```python
from build123d import *

# Parameters (mm, degrees)
SKETCH_1_W             = 80
SKETCH_1_H             = 60
SKETCH_1_W_2           = 78.6
SKETCH_1_H_2           = 58.6
EXTRUDE_1_DEPTH        = 1000
CUT_EXTRUDE_1_REACH    = 1004.597
SKETCH_2_W             = 40
SKETCH_2_H             = 40
PATTERN_LINEAR_1_COUNT = 5
PATTERN_LINEAR_1_PITCH = 200


with BuildPart() as part:
    # 스케치1 → 보스-돌출1 (new body)
    with BuildSketch(Plane.XY):
        Rectangle(SKETCH_1_W, SKETCH_1_H)
        Rectangle(SKETCH_1_W_2, SKETCH_1_H_2, mode=Mode.SUBTRACT)
    extrude(amount=EXTRUDE_1_DEPTH)

    # 스케치2 → 컷-돌출1 (cut, up to next)
    with BuildSketch(Plane(origin=(0, 30, 0), x_dir=(1, 0, 0), z_dir=(0, 1, 0)), mode=Mode.PRIVATE) as cut_extrude_1_sk1:
        with Locations((0, -40)):
            Rectangle(SKETCH_2_W, SKETCH_2_H)
    cut_extrude_1_tool1 = extrude(cut_extrude_1_sk1.sketch, amount=-CUT_EXTRUDE_1_REACH, mode=Mode.PRIVATE) & part.part
    cut_extrude_1 = cut_extrude_1_tool1.solids().sort_by_distance((0, 30, 40))[0]
    add(cut_extrude_1, mode=Mode.SUBTRACT)

    # 선형 패턴1: 컷-돌출1 ×5
    with Locations(*[(0, 0, i * PATTERN_LINEAR_1_PITCH) for i in range(1, PATTERN_LINEAR_1_COUNT)]):
        add(cut_extrude_1, mode=Mode.SUBTRACT)


solid = part.part
```
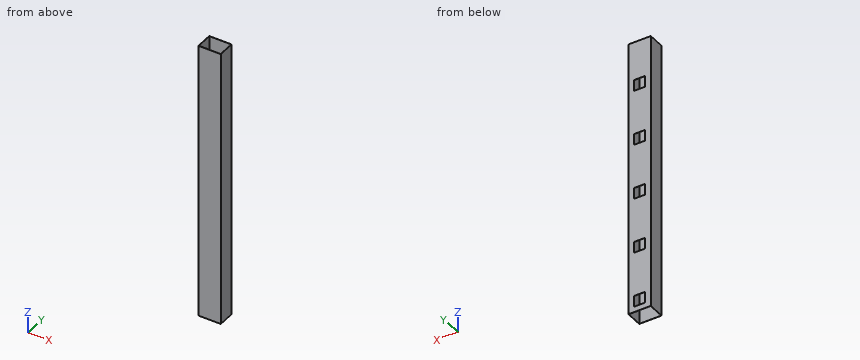
CAD build for the part. Positions are in the model's coordinates, mm. Coordinates: 2 decimals unless noted, no trailing zeros. Order: outer loops, then holes, each group sorted by start corner. A loop starts at its lowest first (then second) coordinate and runs counter-clockwise, first axis right, second up. Notation, with made-up numbers: (15.5, -16) -> (63.5, -16) arc R13 cw to (63.5, -5) -> close; hole circle Ø4 at (-32.5, 23.5). An arc over 180 degrees is marked (long way). Use one line per item in the form item = value. Start each with the question number.
1) Band-saw the part on A-A on z = 100. Give the cut face in (x, y).
2) Band-saw the part on C-C on y = 6.5. Give the cut face in (x, z).
3) Band-saw the part on B-B on x = -29. Give the cut face in (y, z).
4) Drill centre lines: L1, parallel to X at y = -18, z = 303.5; L2, parallel to Y at x = 29, z = 618.5; L3, parallel to Y at x = -14.5, z = 47. Where is each one in solid material? Low to high. Write a range as [from, to].
Entries:
q1.outline = (-40, -30) -> (40, -30) -> (40, 30) -> (-40, 30) -> close; hole (-39.3, -29.3) -> (39.3, -29.3) -> (39.3, 29.3) -> (-39.3, 29.3) -> close
q2.outline = (-40, 0) -> (-39.3, 0) -> (-39.3, 1000) -> (-40, 1000) -> close; (39.3, 0) -> (40, 0) -> (40, 1000) -> (39.3, 1000) -> close
q3.outline = (-30, 0) -> (-29.3, 0) -> (-29.3, 1000) -> (-30, 1000) -> close; (29.3, 0) -> (30, 0) -> (30, 1000) -> (29.3, 1000) -> close
q4.L1 = [-40, -39.3], [39.3, 40]
q4.L2 = [-30, -29.3], [29.3, 30]
q4.L3 = [-30, -29.3]
